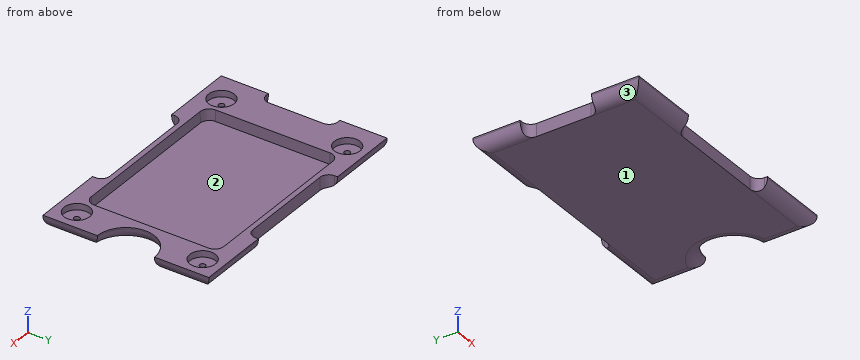
```python
from build123d import *

# Parameters (mm, degrees)
Y_KSEKLIK_EKSTR_ZYON1_DEPTH = 4.5
KES_EKSTR_ZYON2_DEPTH       = 3.9
IZIM7_R                     = 4.5
KES_EKSTR_ZYON3_DEPTH       = 2.2
IZIM9_R                     = 1
KES_EKSTR_ZYON4_DEPTH       = 2
RADYUS4_R                   = 4
PAH1_SIZE                   = 0.2
PAH1_SIZE_2                 = 11.457992326


# Some blends are built 0.0001 mm under size
with BuildPart() as part:
    # Çizim4 → Yükseklik-Ekstrüzyon1 (new body)
    with BuildSketch(Plane.XY):
        with BuildLine():
            Line((200.606144994, -119.46781712), (200.606144994, -100.46781712))
            ThreePointArc((200.606144994, -100.46781712), (190.606144994, -90.46781712), (200.606144994, -80.46781712))
            Line((200.606144994, -80.46781712), (200.606144994, -61.46781712))
            Line((200.606144994, -61.46781712), (175.606144994, -61.46781712))
            Line((175.606144994, -61.46781712), (175.606144994, -62.46781712))
            ThreePointArc((175.606144994, -62.46781712), (174.727465338, -64.589137464), (172.606144994, -65.46781712))
            Line((172.606144994, -65.46781712), (138.606144994, -65.46781712))
            ThreePointArc((138.606144994, -65.46781712), (136.484824651, -64.589137464), (135.606144994, -62.46781712))
            Line((135.606144994, -62.46781712), (135.606144994, -61.46781712))
            Line((135.606144994, -61.46781712), (110.606144994, -61.46781712))
            Line((110.606144994, -61.46781712), (110.606144994, -77.96781712))
            Line((110.606144994, -77.96781712), (111.606144994, -77.96781712))
            ThreePointArc((111.606144994, -77.96781712), (113.727465338, -78.846496777), (114.606144994, -80.96781712))
            Line((114.606144994, -80.96781712), (114.606144994, -99.96781712))
            ThreePointArc((114.606144994, -99.96781712), (113.727465338, -102.089137464), (111.606144994, -102.96781712))
            Line((111.606144994, -102.96781712), (110.606144994, -102.96781712))
            Line((110.606144994, -102.96781712), (110.606144994, -119.46781712))
            Line((110.606144994, -119.46781712), (135.606144994, -119.46781712))
            Line((135.606144994, -119.46781712), (135.606144994, -118.46781712))
            ThreePointArc((135.606144994, -118.46781712), (136.484824651, -116.346496777), (138.606144994, -115.46781712))
            Line((138.606144994, -115.46781712), (172.606144994, -115.46781712))
            ThreePointArc((172.606144994, -115.46781712), (174.727465338, -116.346496777), (175.606144994, -118.46781712))
            Line((175.606144994, -118.46781712), (175.606144994, -119.46781712))
            Line((175.606144994, -119.46781712), (200.606144994, -119.46781712))
        make_face()
    extrude(amount=Y_KSEKLIK_EKSTR_ZYON1_DEPTH)

    # Çizim6 → Kes-Ekstrüzyon2 (cut)
    with BuildSketch(Plane.XY.offset(4.5)):
        with BuildLine():
            Line((129.606144994, -67.46781712), (184.606144994, -67.46781712))
            ThreePointArc((184.606144994, -67.46781712), (186.727465338, -68.346496777), (187.606144994, -70.46781712))
            Line((187.606144994, -70.46781712), (187.606144994, -110.46781712))
            ThreePointArc((187.606144994, -110.46781712), (186.727465338, -112.589137464), (184.606144994, -113.46781712))
            Line((184.606144994, -113.46781712), (129.606144994, -113.46781712))
            ThreePointArc((129.606144994, -113.46781712), (127.484824651, -112.589137464), (126.606144994, -110.46781712))
            Line((126.606144994, -110.46781712), (126.606144994, -70.46781712))
            ThreePointArc((126.606144994, -70.46781712), (127.484824651, -68.346496777), (129.606144994, -67.46781712))
        make_face()
    extrude(amount=-KES_EKSTR_ZYON2_DEPTH, mode=Mode.SUBTRACT)

    # Çizim7 → Kes-Ekstrüzyon3 (cut)
    with BuildSketch(Plane.XY.offset(4.5)):
        with Locations((193.606144994, -68.46781712)):
            Circle(IZIM7_R)
        with Locations((193.606144994, -112.46781712)):
            Circle(IZIM7_R)
        with Locations((120.606144994, -68.46781712)):
            Circle(IZIM7_R)
        with Locations((120.606144994, -112.46781712)):
            Circle(IZIM7_R)
    extrude(amount=-KES_EKSTR_ZYON3_DEPTH, mode=Mode.SUBTRACT)

    # Çizim9 → Kes-Ekstrüzyon4 (cut)
    with BuildSketch(Plane.XY.offset(2.3)):
        with Locations((193.606144994, -68.46781712)):
            Circle(IZIM9_R)
        with Locations((193.606144994, -112.46781712)):
            Circle(IZIM9_R)
        with Locations((120.606144994, -68.46781712)):
            Circle(IZIM9_R)
        with Locations((120.606144994, -112.46781712)):
            Circle(IZIM9_R)
    extrude(amount=-KES_EKSTR_ZYON4_DEPTH, mode=Mode.SUBTRACT)

    # Radyus4
    radyus4_edges = [part.edges().sort_by_distance(p)[0] for p in [
        (123.106144994, -61.46781712, 0),
        (110.606144994, -111.21781712, 0),
        (123.106144994, -119.46781712, 0),
        (188.106144994, -119.46781712, 0),
        (188.106144994, -61.46781712, 0),
        (110.606144994, -69.71781712, 0),
        (200.606144994, -70.96781712, 0),
        (190.606144994, -90.46781712, 0),
        (200.606144994, -109.96781712, 0),
    ]]
    fillet(radyus4_edges, radius=RADYUS4_R - 0.0001)  # a hair under: the kernel refuses the full size

    # Pah1
    # the kernel refuses this chamfer: 11.457992326, 0.2 mm, written as the material it takes off along each edge
    with BuildSketch(Plane(origin=(184.606144994, -70.46781712, 4.5), x_dir=(0, 1, 0), z_dir=(-1, 0, 0))) as pah1_piece_1_section:
        Polygon((3 + PAH1_SIZE, 0), (3, PAH1_SIZE_2), (3, 0), align=None)
    pah1_piece_1 = revolve(axis=Axis((184.606144994, -70.46781712, 4.5), (0, 0, -1)), revolution_arc=90, mode=Mode.PRIVATE)
    pah1_piece_1 = split(pah1_piece_1, bisect_by=Plane(origin=(184.990398639, -67.399868147, 0.6), z_dir=(0, 0, 1)), keep=Keep.TOP, mode=Mode.PRIVATE)
    add(pah1_piece_1, mode=Mode.SUBTRACT)
    with BuildSketch(Plane(origin=(187.606144994, -70.46781712, 4.5), x_dir=(0.41331439412646753, 0, 0.9105883875867686), z_dir=(0, -1, 0))) as pah1_piece_2_section:
        Polygon((PAH1_SIZE * 0.413314394126, -PAH1_SIZE * 0.910588387587), (-PAH1_SIZE_2 * 0.910588387599, -PAH1_SIZE_2 * 0.413314394132), (0, 0), align=None)
    pah1_piece_2 = extrude(amount=40, mode=Mode.PRIVATE)
    pah1_piece_2 = split(pah1_piece_2, bisect_by=Plane(origin=(187.689115858, -74.555184991, 0.6), z_dir=(0, 0, 1)), keep=Keep.TOP, mode=Mode.PRIVATE)
    add(pah1_piece_2, mode=Mode.SUBTRACT)
    with BuildSketch(Plane(origin=(184.606144994, -110.46781712, 4.5), x_dir=(1, 0, 0), z_dir=(0, 1, 0))) as pah1_piece_3_section:
        Polygon((3 + PAH1_SIZE, 0), (3, PAH1_SIZE_2), (3, 0), align=None)
    pah1_piece_3 = revolve(axis=Axis((184.606144994, -110.46781712, 4.5), (0, 0, -1)), revolution_arc=90, mode=Mode.PRIVATE)
    pah1_piece_3 = split(pah1_piece_3, bisect_by=Plane(origin=(187.674093967, -110.852070765, 0.6), z_dir=(0, 0, 1)), keep=Keep.TOP, mode=Mode.PRIVATE)
    add(pah1_piece_3, mode=Mode.SUBTRACT)
    with BuildSketch(Plane(origin=(184.606144994, -113.46781712, 4.5), x_dir=(0, -0.41331439412651433, 0.9105883875867473), z_dir=(-1, 0, 0))) as pah1_piece_4_section:
        Polygon((PAH1_SIZE * 0.413314394127, -PAH1_SIZE * 0.910588387587), (-PAH1_SIZE_2 * 0.910588387599, -PAH1_SIZE_2 * 0.413314394132), (0, 0), align=None)
    pah1_piece_4 = extrude(amount=55, mode=Mode.PRIVATE)
    pah1_piece_4 = split(pah1_piece_4, bisect_by=Plane(origin=(157.106144994, -113.55196189, 0.6), z_dir=(0, 0, 1)), keep=Keep.TOP, mode=Mode.PRIVATE)
    add(pah1_piece_4, mode=Mode.SUBTRACT)
    with BuildSketch(Plane(origin=(129.606144994, -110.46781712, 4.5), x_dir=(0, -1, 0), z_dir=(1, 0, 0))) as pah1_piece_5_section:
        Polygon((3 + PAH1_SIZE, 0), (3, PAH1_SIZE_2), (3, 0), align=None)
    pah1_piece_5 = revolve(axis=Axis((129.606144994, -110.46781712, 4.5), (0, 0, -1)), revolution_arc=90, mode=Mode.PRIVATE)
    pah1_piece_5 = split(pah1_piece_5, bisect_by=Plane(origin=(129.22189135, -113.535766093, 0.6), z_dir=(0, 0, 1)), keep=Keep.TOP, mode=Mode.PRIVATE)
    add(pah1_piece_5, mode=Mode.SUBTRACT)
    with BuildSketch(Plane(origin=(126.606144994, -110.46781712, 4.5), x_dir=(-0.41331439412651433, 0, 0.9105883875867473), z_dir=(0, 1, 0))) as pah1_piece_6_section:
        Polygon((PAH1_SIZE * 0.413314394127, -PAH1_SIZE * 0.910588387587), (-PAH1_SIZE_2 * 0.910588387599, -PAH1_SIZE_2 * 0.413314394132), (0, 0), align=None)
    pah1_piece_6 = extrude(amount=40, mode=Mode.PRIVATE)
    pah1_piece_6 = split(pah1_piece_6, bisect_by=Plane(origin=(126.522000225, -90.46781712, 0.6), z_dir=(0, 0, 1)), keep=Keep.TOP, mode=Mode.PRIVATE)
    add(pah1_piece_6, mode=Mode.SUBTRACT)
    with BuildSketch(Plane(origin=(129.606144994, -70.46781712, 4.5), x_dir=(-1, 0, 0), z_dir=(0, -1, 0))) as pah1_piece_7_section:
        Polygon((3 + PAH1_SIZE, 0), (3, PAH1_SIZE_2), (3, 0), align=None)
    pah1_piece_7 = revolve(axis=Axis((129.606144994, -70.46781712, 4.5), (0, 0, -1)), revolution_arc=90, mode=Mode.PRIVATE)
    pah1_piece_7 = split(pah1_piece_7, bisect_by=Plane(origin=(126.538196021, -70.083563476, 0.6), z_dir=(0, 0, 1)), keep=Keep.TOP, mode=Mode.PRIVATE)
    add(pah1_piece_7, mode=Mode.SUBTRACT)
    with BuildSketch(Plane(origin=(129.606144994, -67.46781712, 4.5), x_dir=(0, 0.41331439412651433, 0.9105883875867473), z_dir=(1, 0, 0))) as pah1_piece_8_section:
        Polygon((PAH1_SIZE * 0.413314394127, -PAH1_SIZE * 0.910588387587), (-PAH1_SIZE_2 * 0.910588387599, -PAH1_SIZE_2 * 0.413314394132), (0, 0), align=None)
    pah1_piece_8 = extrude(amount=55, mode=Mode.PRIVATE)
    pah1_piece_8 = split(pah1_piece_8, bisect_by=Plane(origin=(157.106144994, -67.383672351, 0.6), z_dir=(0, 0, 1)), keep=Keep.TOP, mode=Mode.PRIVATE)
    add(pah1_piece_8, mode=Mode.SUBTRACT)


solid = part.part
```
Geometry check sheet. Reference: the model listing, model coordinates, mm. Face numbers are marked on the shaded views. Round coordinates to 2 decimals unless told otherwise and drop trailing zeros. Loops run counter-clockwise (first coordinate to the right, second up) from the corner with the lowest first, then second, coordinate; pieces in that order, holes last. Notation, with made-up numbers: (-34.75, 74.25) - (-21.75, 74.25) arc R37 ccw to (-21.75, 113.25) - close; hole circle Ø8 at (3, -3.5). An arc over 180 degrees is marked (long way). Write item = value, one per line. Start each with the question number.
1. Thickness scan on line 1 (X direction, y = -112, z = 4); line 2 (X direction, y = -105, z = 3.65); line 3 (Y direction, x = 124, z = 3.9). Record the ranges inside material, lowest first.
2. Depth check by flat-ended pin: pin 1 (1 mm diameter, centred on x = 139, z = 2, fed in from +Y); pin 2 (1.1 mm diameter, centred on y = -62, z = 3, fed in from +X); pin 3 (1.5 mm diameter, centred on x = 172, y = -85, fed in from -Z); pin 4 (1 mm diameter, centred on x = 147, y = -99.5, fed in from +Z). Enter the tip coordinate at first touch or a pass-through.
3. Section check B-B on y = -74.5. Enter the section's corners in (x, z).
4. Mould release check, pull along X, two halves, no side actions. Record for the marked faces 1, 2 and 3: released by +X, released by -X, zero draft, split by the parting line, or undercut.
5. Section check C-C on y = -109.5. Enter the section's corners in (x, z).
6. Section check D-D on x = 124. Enter the section's corners in (y, z), then the cut area to 3 significant figures.
7. Section check A-A on x = 161. Enter the section's corners in (y, z), then the cut area to 3 significant figures.
Working result:
q1.line_1 = 110.61 to 116.13, 125.08 to 126.81, 187.41 to 189.13, 198.08 to 200.61
q1.line_2 = 110.62 to 126.42, 187.79 to 200.59
q1.line_3 = -119.47 to -115.42, -109.51 to -71.42, -65.51 to -61.47
q2.pin_1 = -65.47
q2.pin_2 = 200.58
q2.pin_3 = 0
q2.pin_4 = 0.6
q3.outline = (110.61, 4) arc R4 ccw to (114.61, 0) - (196.61, 0) arc R4 ccw to (200.61, 4) - (200.61, 4.5) - (187.81, 4.5) - (187.74, 0.6) - (126.47, 0.6) - (126.41, 4.5) - (110.61, 4.5) - close
q4.face_1 = zero draft
q4.face_2 = undercut
q4.face_3 = released by -X
q5.outline = (110.61, 4) arc R4 ccw to (114.61, 0) - (196.61, 0) arc R4 ccw to (200.61, 4) - (200.61, 4.5) - (196.99, 4.5) - (196.99, 2.3) - (190.22, 2.3) - (190.22, 4.5) - (187.81, 4.5) - (187.74, 0.6) - (126.47, 0.6) - (126.41, 4.5) - (123.99, 4.5) - (123.99, 2.3) - (117.22, 2.3) - (117.22, 4.5) - (110.61, 4.5) - close
q6.outline = (-119.47, 4) arc R4 ccw to (-115.47, 0) - (-65.47, 0) arc R4 ccw to (-61.47, 4) - (-61.47, 4.5) - (-65.51, 4.5) - (-65.51, 2.3) - (-71.42, 2.3) - (-71.42, 4.5) - (-109.51, 4.5) - (-109.51, 2.3) - (-115.42, 2.3) - (-115.42, 4.5) - (-119.47, 4.5) - close
q6.area = 228 mm^2
q7.outline = (-115.47, 0) - (-65.47, 0) - (-65.47, 4.5) - (-67.27, 4.5) - (-67.34, 0.6) - (-113.6, 0.6) - (-113.67, 4.5) - (-115.47, 4.5) - close
q7.area = 44.3 mm^2
